Part print with two shaded views. Sizes in mm from the minimum x, y, z corner. Round coordinates to 2 decimals unless told otherwise and drop trailing zeros. Order: outer loops, then holes, each group sorted by start corner. A loop starts at its lowest first (then second) coordinate and runs counter-clockwise, first axis right, second up. Notation, with made-up numbers: M -32.75,62.5 L -11.75,62.5 A11 ccw -11.75,81.5 Z; hole C 85.5,-1.75 d7. An arc over 180 degrees is marked long. Return JSON: item names as keys, results as strings. Group by question number.
Item 1: Slice it at D-D on z = 18. Write the cut outline in (x, y), then the cut area to 3 significant figures.
Item 2: Slice it at B-B on z = 30. Write the cut outline in (x, y).
Item 3: Slice it at C-C on x = 6.5. Write the cut outline in (y, z) (1 decimal).
Item 4: Probe line 1 along Y through (x, z) = (2.5, 32) (1 decimal); line 2 along Y through (x, z) = (4, 37.5) (1 decimal); line 3 along Y through (x, z) = (5, 39) (1 decimal). List the from-to ranges inside material, lowest first.
Item 5: Pin check, flat tips, straight feed: pin 1 Ø5 at (x, y) = (6, 73.5) entering from +Z; pin 2 Ø1 at (x, y) = (5.5, 44.5) entering from -Z; pin 3 Ø1 at (x, y) = (4.5, 78.5) entering from +Z; pin 4 Ø7 at (y, z) = (85, 30) entering from -X. Stop position of each tip, or through.
Item 6: Slice it at A-A on y = 50. Write the cut outline in (x, z).
Item 7: Pull direction Z, two halves, no side cores. Call the marked faces 1, 2 and 3: pulls with the +Z half, pulls with the -Z half, needs draft (parallel to the pull), parting line crosses it, or undercut.
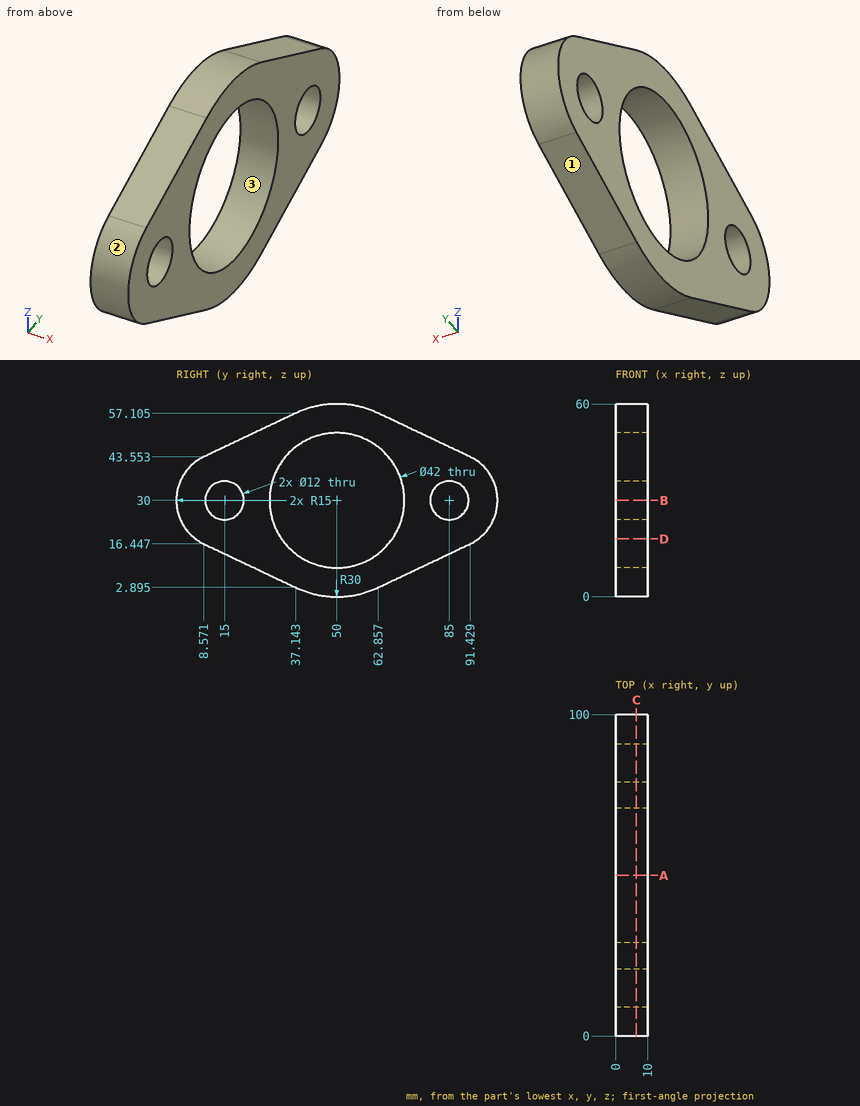
Output values:
{
 "1": {"outline": "M 0,6 L 10,6 L 10,32.77 L 0,32.77 Z; M 0,67.23 L 10,67.23 L 10,94 L 0,94 Z", "area": "535 mm²"},
 "2": {"outline": "M 0,0 L 10,0 L 10,9 L 0,9 Z; M 0,21 L 10,21 L 10,29 L 0,29 Z; M 0,71 L 10,71 L 10,79 L 0,79 Z; M 0,91 L 10,91 L 10,100 L 0,100 Z"},
 "3": {"outline": "M 8.6,16.4 L 37.1,2.9 A30 ccw 62.9,2.9 L 91.4,16.4 A15 ccw 91.4,43.6 L 62.9,57.1 A30 ccw 37.1,57.1 L 8.6,43.6 A15 ccw Z; hole C 15,30 d12; hole C 50,30 d42; hole C 85,30 d12"},
 "4": {"line 1": "0.1 to 9.3, 20.7 to 29.1, 70.9 to 79.3, 90.7 to 99.9", "line 2": "2 to 30.4, 69.6 to 98", "line 3": "3 to 31, 69 to 97"},
 "5": {"pin 1": "z = 53.24", "pin 2": "z = 0.42", "pin 3": "z = 49.92", "pin 4": "through"},
 "6": {"outline": "M 0,0 L 10,0 L 10,9 L 0,9 Z; M 0,51 L 10,51 L 10,60 L 0,60 Z"},
 "7": {"face 1": "pulls with the -Z half", "face 2": "parting line crosses it", "face 3": "undercut"}
}
